Can you work these out from the model? Positions are in its coordinate system, mm. A direction names the side the tool comes from. Give positions to 0.01 mm unless a question says otherwise; leave off trailing zeros. Loops run counter-clockwise (first coordinate to the right, second up) from the corner with the lowest first, then second, coordinate; pieces in that order, holes last. Notation, with made-up numbers: (68.5, 78.5) - (111.5, 78.5) arc R29 cw to (111.5, 115.5) - close; hole circle Ø10 at (-23.5, 6.25). An arc over 180 degrees is marked (long way). Use a Markdown table: item, result. Add a question column.
Autodesk Inventor part; units mm, degrees
ref_plane "YZ Plane" through (0, 0, 0) normal (1, 0, 0) x (0, 1, 0)
ref_plane "XZ Plane" through (0, 0, 0) normal (0, 1, 0) x (-1, 0, 0)
ref_plane "XY Plane" through (0, 0, 0) normal (0, 0, 1) x (1, 0, 0)
sketch "Sketch1" plane through (0, 0, 0) normal (0, 0, 1) x (1, 0, 0)
  line L0 (-29.5815, 53.7121) -> (-29.5815, 355.2879)
  line L1 (-329.5815, 355.5) -> (-54.5815, 355.5)
  line L2 (-329.5815, 53.5) -> (-54.5815, 53.5)
  line L3 (-310.5815, 334.5) -> (-310.5815, 74.5)
  line L4 (-29.5815, 355.5) -> (-310.5815, 355.5)
  line L5 (-310.5815, 355.5) -> (-310.5815, 53.5)
  line L6 (-310.5815, 53.5) -> (-29.5815, 53.5)
  line L7 (-29.5815, 53.5) -> (-29.5815, 355.5)
  point P0 (0, 0)
extrude "Plate1" add sketch "Sketch1" along normal blind 1
sketch "Sketch2" plane through (-29.5815, 53.5, 0) normal (1, 0, 0) x (0, 1, 0)
  line L0 (302, 0) -> (0, 0)
  line L1 (0, 0) -> (0, -21)
  line L2 (0, -21) -> (302, -21)
  line L3 (302, -21) -> (302, 0)
edge flange "Flange1" height 22 angle 90 thickness 1 bend radius 1 thickness toward (1, 0, 0) relief tear relief width 1 relief depth 0.5 edges at (-29.5815, 204.5, 0) wall of the first edge with corners at (-29.5815, 355.5, 0) (-29.5815, 53.5, 0) (-29.5815, 53.5, -21) (-29.5815, 355.5, -21)
bend "Bend1"
corner "Corner1"
chamfer "Corner Chamfer1" distance 18 angle 45 1 edges at (-29.0815, 355.5, -21)
chamfer "Corner Chamfer2" distance 18 angle 45 1 edges at (-29.0815, 53.5, -21)
chamfer "Corner Chamfer3" distance 6 angle 45 2 edges at (-310.5815, 355.5, 0.5) (-310.5815, 53.5, 0.5)
sketch "Sketch3" plane through (0, 0, 1) normal (0, 0, 1) x (1, 0, 0)
  line L0 (-310.5815, 59.5) -> (-310.5815, 349.5)
  line L1 (-304.5815, 355.5) -> (-30.5815, 355.5)
  line L2 (-304.5815, 53.5) -> (-30.5815, 53.5)
  point P0 (0, 0)
  point P1 (-77.5815, 345.5)
  point P2 (-167.5815, 345.5)
  point P3 (-257.5815, 345.5)
  point P4 (-300.5815, 344.5)
  point P5 (-300.5815, 204.5)
  point P6 (-300.5815, 64.5)
  point P7 (-257.5815, 63.5)
  point P8 (-167.5815, 63.5)
  point P9 (-77.5815, 63.5)
  point P10 (-310.5815, 204.5)
  point P11 (-167.5815, 355.5)
  dimension "d20" = 90
  dimension "d21" = 90
  dimension "d22" = 10
  dimension "d23" = 10
  dimension "d24" = 140
  dimension "d25" = 140
  dimension "d26" = 10
hole "Hole1" at (-77.5815, 345.5, 1) at (-167.5815, 345.5, 1) at (-257.5815, 345.5, 1) at (-300.5815, 344.5, 1) at (-300.5815, 204.5, 1) at (-300.5815, 64.5, 1) at (-257.5815, 63.5, 1) at (-167.5815, 63.5, 1) at (-77.5815, 63.5, 1) direction (0, 0, -1) diameter 4 depth 1 tip angle 118
sketch "Sketch4" plane through (-28.5815, 53.5, -1) normal (1, 0, 0) x (0, 0, -1)
  line L0 (20, 284) -> (20, 18)
  point P0 (-1, -53.5)
  point P1 (10, 291)
  point P2 (10, 151)
  point P3 (10, 11)
  point P4 (20, 151)
  dimension "d34" = 10
  dimension "d35" = 140
  dimension "d36" = 140
hole "Hole2" at (-28.5815, 344.5, -11) at (-28.5815, 204.5, -11) at (-28.5815, 64.5, -11) direction (-1, 0, 0) diameter 4 depth 1 tip angle 118
sketch "Sketch5" plane through (0, 0, 1) normal (0, 0, 1) x (1, 0, 0)
  line L0 (-288.5815, 83.5) -> (-288.5815, 325.5)
  line L1 (-329.5815, 74.5) -> (-54.5815, 74.5)
  line L2 (-204.5815, 234.5) -> (-288.5815, 234.5)
  line L3 (-288.5815, 234.5) -> (-288.5815, 74.5)
  line L4 (-288.5815, 74.5) -> (-204.5815, 74.5)
  line L5 (-204.5815, 74.5) -> (-204.5815, 234.5)
  point P0 (0, 0)
  dimension "d44" = 84
  dimension "d45" = 160
extrude "Cut1" cut sketch "Sketch5" against normal blind 1
fillet "Corner Round1" radius 6 4 edges at (-204.5815, 234.5, 0.5) (-288.5815, 234.5, 0.5) (-204.5815, 74.5, 0.5) (-288.5815, 74.5, 0.5)
sketch "Sketch6" plane through (0, 0, 1) normal (0, 0, 1) x (1, 0, 0)
  line L0 (-304.5815, 355.5) -> (-30.5815, 355.5)
  line L1 (-310.5815, 349.5) -> (-310.5815, 59.5)
  point P0 (0, 0)
  point P1 (-280.5815, 325.5)
  dimension "d49" = 30
  dimension "d50" = 30
hole "Hole3" at (-280.5815, 325.5, 1) direction (0, 0, -1) diameter 8 depth 1 tip angle 118
equation "\"d32\" = Thickness"
equation "\"d42\" = Thickness"
equation "\"d46\" = Thickness"
equation "\"d56\" = Thickness"
equation "\"d1\" = BendReliefWidth"
equation "\"d2\" = BendReliefDepth"
equation "\"d3\" = MinimumRemnant"
equation "\"d4\" = BendRadius"
equation "\"d7\" = BendRadius"
equation "\"d8\" = CornerReliefSize"
equation "\"d9\" = GapSize"
equation "\"d10\" = JacobiRadiusSize"
equation "\"BendRadius\" = Thickness"
equation "\"BendReliefWidth\" = Thickness"
equation "\"BendReliefDepth\" = 0.5 * Thickness"
equation "\"CornerReliefSize\" = 4 * Thickness"
equation "\"MinimumRemnant\" = 2 * Thickness"
equation "\"TransitionRadius\" = BendRadius"
equation "\"JacobiRadiusSize\" = BendRadius"
equation "\"GapSize\" = Thickness"
equation "\"d0\" = BendRadius"
properties part number "sheetblack"
1. Please list where these lines run through material, in increasing order: line 1 along Y through (x, z) = (-29.3, -11); line 2 along X through (y, z) = (63.5, 0.7); line 3 along X through (y, z) = (278, -10.5). Write a range as [from, to].
2. Suppose I cut it at A-A (y = 325.5). List the corners of the cut face in (x, z) for me.
3. Will these pins go through, and if not, where does the flat tip stop? P1, Ø1.5, axis at x = -261.5, y = 254.5, coming from the -Z side; P2, Ø6.5, axis at x = -300.58, y = 204.5, coming from the +Z side; P3, Ø1.1, axis at y = 152, z = 0.5, coming from the +X side; P4, Ø4, axis at y = 133.5, z = -16, coming from the -X side.
4. Suppose I cut it at B-B (x = -266). List the corners of the cut face in (y, z) for me, and give its area (3 significant figures).
5. On a 3-axis mill with a long thin cutter (end or side, diameter ignored), from which of +Z, -Z, +X, -X, +Y, -Y can I reach the whole of each face in a straight line? I mean faces 1 (the face through (-29.1, 346.4, -12.1)), 2 (the face through (-173, 207, 0)). Say none if no direction works.
6. Suppose I cut it at C-C (y = 193.5). List the corners of the cut face in (x, z) for me.
7. Suppose I cut it at D-D (x = -128). List the corners of the cut face in (y, z) for me.
Results below:
| question | item | result |
|---|---|---|
| 1 | line 1 | [61.5, 62.5], [66.5, 202.5], [206.5, 342.5], [346.5, 347.5] |
| 1 | line 2 | [-310.58, -302.31], [-298.85, -259.58], [-255.58, -169.58], [-165.58, -79.58], [-75.58, -29.53] |
| 1 | line 3 | [-29.58, -28.58] |
| 2 | outline | (-310.58, 0) - (-284.58, 0) - (-284.58, 1) - (-310.58, 1) - close; (-276.58, 0) - (-30.58, 0) arc R1 cw to (-29.58, -1) - (-29.58, -21) - (-28.58, -21) - (-28.58, -1) arc R2 ccw to (-30.58, 1) - (-276.58, 1) - close |
| 3 | P1 | z = 0 |
| 3 | P2 | z = 1 |
| 3 | P3 | x = -28.82 |
| 3 | P4 | x = -29.58 |
| 4 | outline | (53.5, 0) - (74.5, 0) - (74.5, 1) - (53.5, 1) - close; (234.5, 0) - (355.5, 0) - (355.5, 1) - (234.5, 1) - close |
| 4 | area | 142 mm² |
| 5 | face 1 | -Z, +X, -X, +Y |
| 5 | face 2 | -Z, -X, +Y, -Y |
| 6 | outline | (-310.58, 0) - (-288.58, 0) - (-288.58, 1) - (-310.58, 1) - close; (-204.58, 0) - (-30.58, 0) arc R1 cw to (-29.58, -1) - (-29.58, -21) - (-28.58, -21) - (-28.58, -1) arc R2 ccw to (-30.58, 1) - (-204.58, 1) - close |
| 7 | outline | (53.5, 0) - (355.5, 0) - (355.5, 1) - (53.5, 1) - close |
